Model file for the job. Use its own axes, mm. Face numbers are marked on the shaded views. A direction names the side the tool comes from. Round coordinates to 2 decimals unless told otherwise and drop trailing zeros. Order: outer loops, then holes, each group sorted by start corner. A loop starts at its lowest first (then second) coordinate and runs counter-clockwise, first axis right, second up. Notation, with made-up numbers: (40.25, 57) - (69.25, 57) arc R11 cw to (69.25, 78) - close; hole circle Ø8 at (80.5, 51.25). An arc over 180 degrees is marked (long way). Write item = value, one per line.
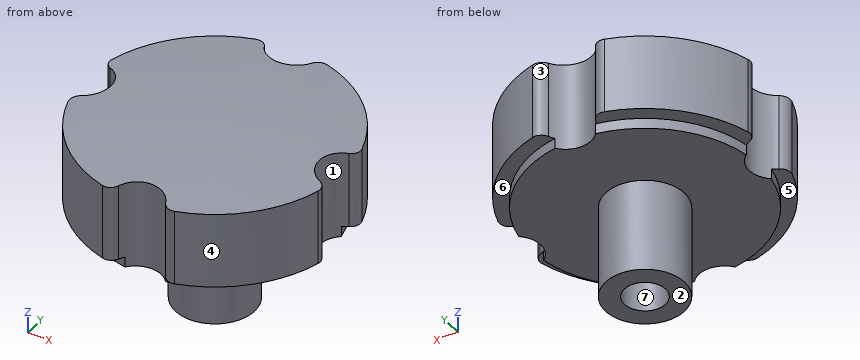
```python
from build123d import *

# Parameters (mm, degrees)
CUT_EXTRUDE1_REACH = 77.517
SKETCH2_R          = 7.5
FILLET1_R          = 3


with BuildPart() as part:
    # Sketch1 → Revolve1 (revolve)
    with BuildSketch(Plane(origin=(0, 0, 0), x_dir=(1, 0, 0), z_dir=(0, 1, 0))):
        with BuildLine():
            Line((0, 23.761691948), (0, 0))
            ThreePointArc((0, 0), (-18.770678987, 0.44066572), (-37.5, 1.761691948))
            Line((-37.5, 1.761691948), (-37.5, 23.761691948))
            Line((-37.5, 23.761691948), (-33.34, 23.761691948))
            Line((-33.34, 23.761691948), (-33.34, 26.761691948))
            Line((-33.34, 26.761691948), (-11.5, 26.761691948))
            Line((-11.5, 26.761691948), (-11.5, 53.761691948))
            Line((-11.5, 53.761691948), (-6, 53.761691948))
            Line((-6, 53.761691948), (-6, 23.761691948))
            Line((-6, 23.761691948), (0, 23.761691948))
        make_face()
    revolve(axis=Axis((0, 0, -358.843484937), (0, 0, 1)))

    # Sketch2 → Cut-Extrude1 (cut, up to next)
    with BuildSketch(Plane.XY, mode=Mode.PRIVATE) as cut_extrude1_sk1:
        with Locations((0, 37.5)):
            Circle(SKETCH2_R)
    cut_extrude1_tool1 = extrude(cut_extrude1_sk1.sketch, amount=-CUT_EXTRUDE1_REACH, mode=Mode.PRIVATE) & part.part
    # Sketch2 → Cut-Extrude1 (cut, up to next)
    with BuildSketch(Plane.XY, mode=Mode.PRIVATE) as cut_extrude1_sk2:
        with Locations((37.5, 0)):
            Circle(SKETCH2_R)
    cut_extrude1_tool2 = extrude(cut_extrude1_sk2.sketch, amount=-CUT_EXTRUDE1_REACH, mode=Mode.PRIVATE) & part.part
    # Sketch2 → Cut-Extrude1 (cut, up to next)
    with BuildSketch(Plane.XY, mode=Mode.PRIVATE) as cut_extrude1_sk3:
        with Locations((0, -37.5)):
            Circle(SKETCH2_R)
    cut_extrude1_tool3 = extrude(cut_extrude1_sk3.sketch, amount=-CUT_EXTRUDE1_REACH, mode=Mode.PRIVATE) & part.part
    # Sketch2 → Cut-Extrude1 (cut, up to next)
    with BuildSketch(Plane.XY, mode=Mode.PRIVATE) as cut_extrude1_sk4:
        with Locations((-37.5, 0)):
            Circle(SKETCH2_R)
    cut_extrude1_tool4 = extrude(cut_extrude1_sk4.sketch, amount=-CUT_EXTRUDE1_REACH, mode=Mode.PRIVATE) & part.part
    add(cut_extrude1_tool1.solids().sort_by_distance((0, 37.5, 0))[0], mode=Mode.SUBTRACT)
    add(cut_extrude1_tool2.solids().sort_by_distance((37.5, 0, 0))[0], mode=Mode.SUBTRACT)
    add(cut_extrude1_tool3.solids().sort_by_distance((0, -37.5, 0))[0], mode=Mode.SUBTRACT)
    add(cut_extrude1_tool4.solids().sort_by_distance((-37.5, 0, 0))[0], mode=Mode.SUBTRACT)

    # Fillet1
    # the kernel refuses this fillet: 3 mm, written as the material it takes off along each edge
    with BuildSketch(Plane(origin=(-36.75, -7.462405778, -31.291256689), x_dir=(0.9654419045574989, 0.26061835876313283, 0), z_dir=(0, 0, 1))) as fillet1_piece_1:
        with BuildLine():
            CenterArc((2.929820443, -2.959993207), FILLET1_R, 99.367586043, 81.606967112)
            ThreePointArc((-0.0697456, -3.01101823), (-0.065113873, -1.504808627), (0, 0))
            ThreePointArc((0, 0), (1.220758518, -0.100016984), (2.441517036, 0))
        make_face()
    extrude(amount=37.059130081, mode=Mode.SUBTRACT)
    with BuildSketch(Plane(origin=(-36.75, 7.462405778, -31.291256689), x_dir=(0.9654419045574933, -0.26061835876315326, 0), z_dir=(0, 0, 1))) as fillet1_piece_2:
        with BuildLine():
            CenterArc((2.929820443, 2.959993207), FILLET1_R, 179.025446846, 81.606967112)
            ThreePointArc((-0.0697456, 3.01101823), (-0.065113873, 1.504808627), (0, 0))
            ThreePointArc((0, 0), (1.220758518, 0.100016984), (2.441517036, 0))
        make_face()
    extrude(amount=37.059129481, mode=Mode.SUBTRACT)
    with BuildSketch(Plane(origin=(7.462405778, -36.75, -31.291256689), x_dir=(-0.26061835876313594, 0.9654419045574982, 0), z_dir=(0, 0, 1)), Plane(origin=(36.75, 7.462405778, -31.291256689), x_dir=(-0.9654419045574977, -0.2606183587631379, 0), z_dir=(0, 0, 1)), Plane(origin=(-7.462405778, 36.75, -31.291256689), x_dir=(0.2606183587631421, -0.9654419045574966, 0), z_dir=(0, 0, 1))) as fillet1_piece_3:
        with BuildLine():
            CenterArc((2.929820443, -2.959993207), FILLET1_R, 99.367586043, 81.606967112)
            ThreePointArc((-0.0697456, -3.01101823), (-0.065113873, -1.504808627), (0, 0))
            ThreePointArc((0, 0), (1.220758518, -0.100016984), (2.441517036, 0))
        make_face()
    extrude(amount=37.059129481, mode=Mode.SUBTRACT)
    with BuildSketch(Plane(origin=(-7.462405778, -36.75, -31.291256689), x_dir=(-0.9712182108388207, 0.238191492155031, 0), z_dir=(0, 0, 1)), Plane(origin=(36.75, -7.462405778, -31.291256689), x_dir=(-0.23819149215502627, -0.9712182108388219, 0), z_dir=(0, 0, 1)), Plane(origin=(7.462405778, 36.75, -31.291256689), x_dir=(0.9712182108388221, -0.2381914921550248, 0), z_dir=(0, 0, 1))) as fillet1_piece_4:
        with BuildLine():
            CenterArc((2.89135286, -2.997580065), FILLET1_R, 87.69851564, 81.606967112)
            ThreePointArc((-0.056538816, -2.440862306), (0.071720755, -1.222747271), (0, 0))
            ThreePointArc((0, 0), (1.505912948, 0.030249184), (3.011825896, 0))
        make_face()
    extrude(amount=37.059129481, mode=Mode.SUBTRACT)


solid = part.part
```
1) Cut at D-D (x = 13.5). Write the cut outline in (y, z).
Conclusion:
outline = (-34.99, -23.76) - (-30.48, -23.76) - (-30.48, -26.76) - (30.48, -26.76) - (30.48, -23.76) - (34.99, -23.76) - (34.99, -1.76) arc R399.77 ccw to (-34.99, -1.76) - close
2) Wall check: line 1 along Y through (x, z) = (0, -40); line 2 along Y through (x, z) = (33.5, -9.5). Give the ranges that are in metal, low to high.
Conclusion:
line_1 = -11.5 to -6, 6 to 11.5
line_2 = -16.85 to -6.34, 6.34 to 16.85
3) 3-axis set-ups, long thin cutter, end or side, ignore diameter. For the marked faces 5, 6 and 7: which of +Z, -Z, +X, -X, +Y, -Y reach the whole face in a straight line?
Conclusion:
face_5 = -Z, -X, -Y
face_6 = -Z, +X, +Y
face_7 = -Z
4) Cut at B-B (x = 0). Write the cut outline in (y, z), and give its area (3 significant figures).
Conclusion:
outline = (-30, -26.76) - (-11.5, -26.76) - (-11.5, -53.76) - (-6, -53.76) - (-6, -23.76) - (6, -23.76) - (6, -53.76) - (11.5, -53.76) - (11.5, -26.76) - (30, -26.76) - (30, -1.13) arc R400 ccw to (-30, -1.13) - close
area = 1,840 mm^2
5) Flat gauge pins, fed straight in: pin 1 Ø10 at (x, z) = (19.5, -18.5) entering from +Y; pin 2 Ø15 at (x, y) = (-24, -28.5) entering from -Z; pin 3 Ø2 at (x, z) = (24.5, -21.5) entering from -Y. Where does each tip first touch, or does it go through?
Conclusion:
pin_1 = 34.58
pin_2 = -26.76
pin_3 = -29.22
6) Cut at A-A (z = -29). Write the cut outline in (x, y), and give its area (3 significant figures).
Conclusion:
outline = circle Ø23 at (0, 0); hole circle Ø12 at (0, 0)
area = 302 mm^2
7) Mould opens along Y. For the marked faces 1, 2, 3 and 4 say: +Y half, -Y half, draft (parallel to the pull), parting line (faces both ways), or undercut.
Conclusion:
face_1 = undercut
face_2 = draft
face_3 = +Y half
face_4 = -Y half
